Part model, mm, in its own coordinate system. A direction names the side the tool comes from. Give positions to 0.01 mm unless a question says otherwise; leave off trailing zeros. Write each loop counter-clockwise with the first axis right and the second up, starting at its lowest first coordinate (ties: lowest second). Pieces come first, ordered by that corner, then holes.
from build123d import *

# Parameters (mm, degrees)
BOSS_EXTRUDE1_DEPTH     = 3.175
SKETCH2_W               = 6.35
SKETCH2_H               = 25.4
BOSS_EXTRUDE2_DEPTH     = 50.8
SKETCH3_R               = 5.207
CUT_EXTRUDE1_DEPTH      = 34.655
CUT_EXTRUDE1_DEPTH_BACK = 297.545


with BuildPart() as part:
    # Sketch1 → Boss-Extrude1 (new body, symmetric)
    with BuildSketch(Plane(origin=(0, 0, 0), x_dir=(1, 0, 0), z_dir=(0, 1, 0))):
        Polygon((161.925, -69.85), (121.92, -69.85), (121.92, -63.5), (106.68, -63.5), (106.68, -69.85), (-106.68, -69.85), (-110.5408, -69.85), (-110.5408, -38.1), (-135.9408, -38.1), (-135.9408, -69.85), (-161.925, -69.85), (-161.925, -34.874677354), (-165.1, -34.874677354), (-165.1, -14.046677354), (-161.925, -14.046677354), (-161.925, -10.414), (-141.605, -10.414), (-141.605, 10.414), (-161.925, 10.414), (-161.925, 14.046677354), (-165.1, 14.046677354), (-165.1, 34.874677354), (-161.925, 34.874677354), (-161.925, 69.85), (-136.779, 69.85), (-136.779, 38.1), (-111.379, 38.1), (-111.379, 69.85), (-22.228595254, 69.85), (-22.228595254, 44.45), (22.228595254, 44.45), (22.228595254, 69.85), (111.379, 69.85), (111.379, 38.1), (136.779, 38.1), (136.779, 69.85), (161.925, 69.85), (161.925, 34.874677354), (165.1, 34.874677354), (165.1, 14.046677354), (161.925, 14.046677354), (161.925, 10.414), (141.605, 10.414), (141.605, -10.414), (161.925, -10.414), (161.925, -14.046677354), (165.1, -14.046677354), (165.1, -34.874677354), (161.925, -34.874677354), align=None)
    extrude(amount=BOSS_EXTRUDE1_DEPTH, both=True)

    # Sketch2 → Boss-Extrude2 (add, symmetric)
    with BuildSketch(Plane(origin=(0, 0, 0), x_dir=(1, 0, 0), z_dir=(0, 1, 0))):
        with Locations((128.27, 0)):
            Rectangle(SKETCH2_W, SKETCH2_H)
        with Locations((-128.27, 0)):
            Rectangle(SKETCH2_W, SKETCH2_H)
    extrude(amount=BOSS_EXTRUDE2_DEPTH, both=True)

    # Sketch3 → Cut-Extrude1 (cut, two sides)
    with BuildSketch(Plane.ZY.offset(131.445)) as cut_extrude1_sk:
        with Locations((0, 43.18)):
            Circle(SKETCH3_R)
        with Locations((0, -43.18)):
            Circle(SKETCH3_R)
    extrude(amount=CUT_EXTRUDE1_DEPTH, mode=Mode.SUBTRACT)
    extrude(cut_extrude1_sk.sketch, amount=-CUT_EXTRUDE1_DEPTH_BACK, mode=Mode.SUBTRACT)


solid = part.part
1) Saw through at D-D (x = -97). Write the cut outline in (y, z) (3 decimals), and give its area (3 significant figures).
Check result:
outline: (-3.175, -69.85) - (3.175, -69.85) - (3.175, 69.85) - (-3.175, 69.85) - close
area: 887 mm2
2) Mould opens along X. For faces 1 (the flat face through (-136.779, 0, -54)), 2 (the cylindrical face through (-128.314, -48.263, -1.129)), 3 (the flat face through (-131.445, 27, 0)), 4 (the flat face through (114, 0, 63.5)) say: +X half, -X half, draft (parallel to the pull), parting line (faces both ways), or undercut.
Check result:
face 1: undercut
face 2: draft
face 3: -X half
face 4: undercut
3) Saw through at C-C (y = 8). Write the cut outline in (x, z) (3 decimals), and give its area (3 significant figures).
Check result:
outline: (-131.445, -12.7) - (-125.095, -12.7) - (-125.095, 12.7) - (-131.445, 12.7) - close; (125.095, -12.7) - (131.445, -12.7) - (131.445, 12.7) - (125.095, 12.7) - close
area: 323 mm2
4) Saw through at B-B (z = 59.5). Write the cut outline in (x, y) (3 decimals).
Check result:
outline: (-161.925, -3.175) - (-135.941, -3.175) - (-135.941, 3.175) - (-161.925, 3.175) - close; (-110.541, -3.175) - (161.925, -3.175) - (161.925, 3.175) - (-110.541, 3.175) - close
5) 3-axis set-ups, long thin cutter, end or side, ignore diameter. For faces 5 (the flat face through (128, -27, 12.7)), 6 (the flat face through (22.229, 0, -57)), 7 (the flat face through (-125.095, 27, 0)), 8 (the flat face through (-128, 27, -12.7)): which of +Z, -Z, +X, -X, +Y, -Y reach the whole face in a straight line?
Check result:
face 5: +Z, +X, -X, -Y
face 6: -Z, +Y, -Y
face 7: +Z, -Z, +Y
face 8: -Z, +X, -X, +Y
6) Drill centre lines: L1, parallel to Y at x = 129, z = 0; L2, parallel to Z at x = 128, y = 43; L3, parallel to X at y = -20.5, z = -8 (3 decimals). Where is each one in solid material? Low to high.
Check result:
L1: y = -50.8 to -48.39, -37.97 to 37.97, 48.39 to 50.8
L2: z = -12.7 to -5.2, 5.2 to 12.7
L3: x = -131.445 to -125.095, 125.095 to 131.445
7) Saw through at A-A (y = -43.18). Write the cut outline in (x, z) (3 decimals).
Check result:
outline: (-131.445, -12.7) - (-125.095, -12.7) - (-125.095, -5.207) - (-131.445, -5.207) - close; (-131.445, 5.207) - (-125.095, 5.207) - (-125.095, 12.7) - (-131.445, 12.7) - close; (125.095, -12.7) - (131.445, -12.7) - (131.445, -5.207) - (125.095, -5.207) - close; (125.095, 5.207) - (131.445, 5.207) - (131.445, 12.7) - (125.095, 12.7) - close
8) Flat gauge pins, fed straight in: P1, Ø1.9, axis at y = -1, z = 0.5, coming from the +X side (3 decimals); P2, Ø1.6, axis at x = 164, y = 0, coming from the -Z side; P3, Ø4, axis at x = 72.5, z = -12.5, coming from the -Y side (3 decimals). Where does each tip first touch, or does it go through?
Check result:
P1: stops at x = 141.605
P2: stops at z = -34.87
P3: stops at y = -3.175
